from build123d import *

# Parameters (mm, degrees)
F1_DEPTH = 5
F3_DEPTH = 12.5
F5_DEPTH = 4.85


with BuildPart() as f1:
    # F0 (on Top) → F1 (new body)
    with BuildSketch(Plane.XY):
        Polygon((-2.800149, 4.85), (-5.600298, 0), (-2.800149, -4.85), (2.800149, -4.85), (5.600298, 0), (2.800149, 4.85), align=None)
        with BuildLine():
            ThreePointArc((-1.204326, -1.235), (0, 1.725), (1.204326, -1.235))
            Line((1.204326, -1.235), (-1.204326, -1.235))
        make_face(mode=Mode.SUBTRACT)
    extrude(amount=F1_DEPTH)

    # F2 (on Right) → F3 (cut, symmetric)
    with BuildSketch(Plane.YZ):
        Polygon((4.85, 3.973057), (4.85, 4.75), (4.461528, 4.361528), align=None)
    extrude(amount=F3_DEPTH, both=True, mode=Mode.SUBTRACT)

    # F4 (on face) → F5 (cut, through all)
    with BuildSketch(Plane.XZ.offset(4.85)):
        with BuildLine():
            ThreePointArc((1.147153, 4.138304), (0, 4.5), (-1.147153, 4.138304))
            ThreePointArc((-1.147153, 4.138304), (0, 0.5), (1.147153, 4.138304))
        make_face()
    extrude(amount=-F5_DEPTH, mode=Mode.SUBTRACT)


solid = f1.part
The listing builds one solid part. Answer for the finished solid, in the listing's coordinates (mm). A direction names the side the tool comes from. Give positions to 0.01 mm unless a question says otherwise; leave off trailing zeros. Loops run counter-clockwise (first coordinate to the right, second up) from the corner with the lowest first, then second, coordinate; pieces in that order, holes last. Notation, with made-up numbers: (54, 20) - (87, 20) arc R22 cw to (87, 49) - close; hole circle Ø7 at (79, 89). An arc over 180 degrees is marked (long way). Answer as a JSON object with one key per item and string values.
1. For faces 4 (the flat face through (0, -1.235, 4.7)), 5 (the flat face through (0, 2, 0)), determine the directions among +Z, -Z, +X, -X, +Y, -Y from which every point of the face is accessible in a straight line to the end or side of a thin tool.
Determined:
{"face 4": "+Z, -Z", "face 5": "-Z, +X, -X, +Y, -Y"}
2. Flat-ended cylindrical pins translate along their axes: pin 1 Ø1 at (x, y) = (-4, 2.5) entering from -Z; pin 2 Ø1 at (y, z) = (3, 2.5) entering from -X; pin 3 Ø3 at (x, z) = (0, 2.5) entering from -Y. Find the tip coordinate at first contact, or state that the pin passes through.
Determined:
{"pin 1": "z = 0", "pin 2": "x = -4.16", "pin 3": "y = 0.85"}
3. A cutting plane is placed at A-A (x = 0). Write down the section's boundary in (y, z) (3 decimals).
Determined:
{"outline": "(-4.85, 0) - (-1.235, 0) - (-1.235, 0.5) - (-4.85, 0.5) - close; (-4.85, 4.5) - (-1.235, 4.5) - (-1.235, 5) - (-4.85, 5) - close; (1.725, 0) - (4.85, 0) - (4.85, 3.973) - (4.462, 4.362) - (4.85, 4.75) - (4.85, 5) - (1.725, 5) - close"}
4. A cutting plane is placed at D-D (y = -2.5). Write down the section's boundary in (x, z).
Determined:
{"outline": "(-4.16, 0) - (4.16, 0) - (4.16, 5) - (-4.16, 5) - close; hole circle Ø4 at (0, 2.5)"}
5. For a pull along X with two mould halves and no side action, classify faces 1 (the cylindrical face through (-0.057, 1.724, 2.465)), 2 (the flat face through (4.18, -2.46, 2.46)), 3 (the flat face through (-2, -4.85, 1)) as pulls with the +X half, pulls with the -X half, needs draft (parallel to the pull), parting line crosses it, or undercut.
Determined:
{"face 1": "undercut", "face 2": "pulls with the +X half", "face 3": "needs draft"}
6. Find the intervals of material crossed by L1, parallel to Z at x = 0, y = -1.8; L2, parallel to X at y = -0.25, z = 4.2; L3, parallel to X at y = -0.95, z = 2.5, in increasing order. Write a range as [from, to].
Determined:
{"L1": "[0, 0.5], [4.5, 5]", "L2": "[-5.46, -1.71], [1.71, 5.46]", "L3": "[-5.05, -2], [2, 5.05]"}
7. A cutting plane is placed at B-B (y = 0.5). Write down the section's boundary in (x, z).
Determined:
{"outline": "(-5.31, 0) - (-1.65, 0) - (-1.65, 5) - (-5.31, 5) - close; (1.65, 0) - (5.31, 0) - (5.31, 5) - (1.65, 5) - close"}
8. A cutting plane is placed at C-C (z = 2.5). Write down the section's boundary in (x, y) (3 decimals), then the cut area to 3 significant figures.
Determined:
{"outline": "(-5.6, 0) - (-2.8, -4.85) - (-2, -4.85) - (-2, 0) - (-1.725, 0) arc R1.725 cw to (1.725, 0) - (2, 0) - (2, -4.85) - (2.8, -4.85) - (5.6, 0) - (2.8, 4.85) - (-2.8, 4.85) - close", "area": "57.4 mm²"}
